from build123d import *

# Parameters (mm, degrees)
SKETCH_1_W          = 50
SKETCH_1_H          = 8
EXTRUDE_1_DEPTH     = 8
SKETCH_2_R          = 2
CUT_EXTRUDE_1_DEPTH = 8
SKETCH_3_W          = 20
SKETCH_3_H          = 8
EXTRUDE_2_DEPTH     = 1
SKETCH_4_R          = 2.25
CUT_EXTRUDE_2_DEPTH = 10
SKETCH_4_3_R        = 2.25
CUT_EXTRUDE_3_DEPTH = 10
CHAMFER_1_SIZE      = 2
CHAMFER_2_SIZE      = 1
CHAMFER_3_SIZE      = 1


with BuildPart() as part:
    # Sketch 1 → Extrude 1 (new body)
    with BuildSketch(Plane.XY):
        Polygon((0, 0), (25, 0), (25, 5), (-25, 5), (-25, 0), align=None)
        Polygon((0, 5), (10, 5), (10, 39), (-10, 39), (-10, 5), align=None)
        with Locations((0, 43)):
            Rectangle(SKETCH_1_W, SKETCH_1_H)
    extrude(amount=-EXTRUDE_1_DEPTH)

    # Sketch 2 → Cut-Extrude 1 (cut)
    with BuildSketch(Plane(origin=(0, 5, 0), x_dir=(1, 0, 0), z_dir=(0, 1, 0))):
        with Locations(Location((19, 4, 0), (0, 0, 180))):
            Circle(SKETCH_2_R)
        with Locations(Location((-19, 4, 0), (0, 0, 180))):
            Circle(SKETCH_2_R)
    extrude(amount=-CUT_EXTRUDE_1_DEPTH, mode=Mode.SUBTRACT)

    # Sketch 3 → Extrude 2 (add)
    with BuildSketch(Plane.XY):
        with Locations((0, 35)):
            Rectangle(SKETCH_3_W, SKETCH_3_H)
    extrude(amount=EXTRUDE_2_DEPTH)

    # Sketch 4 → Cut-Extrude 2 (cut)
    with BuildSketch(Plane(origin=(0, 47, 0), x_dir=(1, 0, 0), z_dir=(0, 1, 0))):
        with Locations(Location((19, 3.847406514, 0), (0, 0, 180))):
            Circle(SKETCH_4_R)
    extrude(amount=-CUT_EXTRUDE_2_DEPTH, mode=Mode.SUBTRACT)

    # Sketch 4_3 → Cut-Extrude 3 (cut)
    with BuildSketch(Plane(origin=(0, 47, 0), x_dir=(1, 0, 0), z_dir=(0, 1, 0))):
        with Locations(Location((19, 3.847406514, 0), (0, 0, 180))):
            Circle(SKETCH_4_3_R)
        with Locations(Location((-19, 3.847406514, 0), (0, 0, 180))):
            Circle(SKETCH_4_3_R)
    extrude(amount=-CUT_EXTRUDE_3_DEPTH, mode=Mode.SUBTRACT)

    # Chamfer 1
    chamfer_1_edges = [part.edges().sort_by_distance(p)[0] for p in [
        (-10, 39, -4),
        (10, 39, -4),
        (10, 5, -4),
        (-10, 5, -4),
    ]]
    chamfer(chamfer_1_edges, length=CHAMFER_1_SIZE)

    # Chamfer 2
    chamfer_2_edges = [part.edges().sort_by_distance(p)[0] for p in [
        (0, 47, 0),
    ]]
    chamfer(chamfer_2_edges, length=CHAMFER_2_SIZE)

    # Chamfer 3
    chamfer_3_edges = [part.edges().sort_by_distance(p)[0] for p in [
        (0, 0, -8),
    ]]
    chamfer(chamfer_3_edges, length=CHAMFER_3_SIZE)


solid = part.part
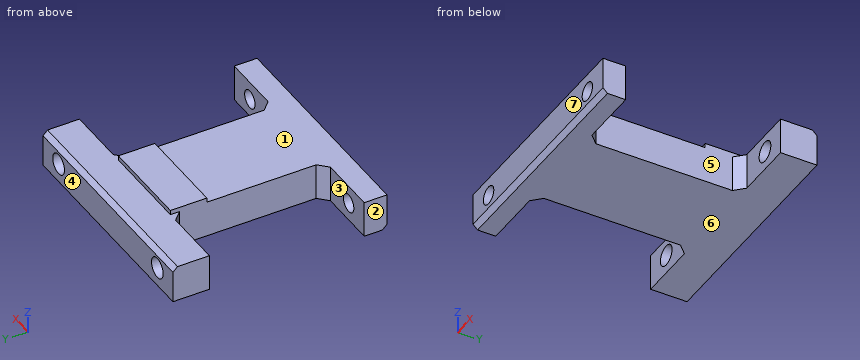
Design review of the part built by this model. Coordinates are the model's own, in mm. Face numbers are marked on the shaded views. A direction names the side the tool comes from. Give positions to 0.01 mm unless a question says otherwise; leave off trailing zeros. Loops run counter-clockwise (first coordinate to the right, second up) from the corner with the lowest first, then second, coordinate; pieces in that order, holes last. Notation, with made-up numbers: M 44.25,69 L 61.25,69 A27 ccw 61.25,98 Z; hole C 20.5,39.5 d5. An arc over 180 degrees is marked long. Answer as a JSON object with one key per item and string values.
Item 1: Mouldability with a two-part tool opening along Y and no side actions: class the marked faces 4, 5, 6 and 7 as pulls with the +Y half, pulls with the -Y half, needs draft (parallel to the pull), parting line crosses it, or undercut.
Output values:
{"face 4": "pulls with the +Y half", "face 5": "undercut", "face 6": "needs draft", "face 7": "pulls with the -Y half"}
Item 2: We need section C-C (z = -5). Count the separate pieces of the cut face and the enclosed holes in it, and give its area (3 significant figures).
Output values:
{"separate pieces": "5", "enclosed holes": "0", "area": "1,240 mm2"}
Item 3: Wall thickness on line 1 along Y through (x, z) = (-22, -5.5); line 2 along Z through (x, y) = (-19, 42.25); line 3 along Z through (x, y) = (19, 1.75): over which ranges is each line inside the solid? List them lowest first.
Output values:
{"line 1": "y = 0 to 5, 39 to 47", "line 2": "z = -8 to -6.1, -1.6 to 0", "line 3": "z = -8 to -6, -2 to 0"}
Item 4: For P1, Ø4, axis at x = 3.5, y = 18, coming from the +Z side; P2, Ø0.5, axis at x = -0.5, z = 0.5, coming from the +Y side; P3, Ø4.5, axis at y = 22, z = -4.5, coming from the -X side, all flat-tipped, find the tip position at first contact; note any pin that passes through.
Output values:
{"P1": "stops at z = 0", "P2": "stops at y = 39", "P3": "stops at x = -10"}
Item 5: Machinability: for the marked faces 1, 2 and 3, which of the approach directions +Z, -Z, +X, -X, +Y, -Y give a long, thin tool a straight path to every point of the face, cutting with its end or side? Answer none if there is none.
Output values:
{"face 1": "+Z, +X, -X, -Y", "face 2": "+Z, -Z, -X, +Y, -Y", "face 3": "+Z, -Z, -X"}
Item 6: We need section D-D (y = 15). State the section outline as (x, z) points.
Output values:
{"outline": "M -10,-8 L 10,-8 L 10,0 L -10,0 Z"}
Item 7: We need section A-A (x = -19). State the section outline as (y, z) points.
Output values:
{"outline": "M 0,-7 L 1,-8 L 5,-8 L 5,-6 L 0,-6 Z; M 0,-2 L 5,-2 L 5,0 L 0,0 Z; M 39,-8 L 47,-8 L 47,-6.1 L 39,-6.1 Z; M 39,-1.6 L 47,-1.6 L 47,-1 L 46,0 L 39,0 Z"}
Item 8: We need section B-B (x = -4). State the section outline as (y, z) points, and give its area (3 significant figures).
Output values:
{"outline": "M 0,-7 L 1,-8 L 47,-8 L 47,-1 L 46,0 L 39,0 L 39,1 L 31,1 L 31,0 L 0,0 Z", "area": "383 mm2"}
